```python
from build123d import *

# Parameters (mm, degrees)
SKETCH1_W           = 60
SKETCH1_H           = 7.9
BOSS_EXTRUDE1_DEPTH = 0.5
SKETCH2_W           = 2.6
SKETCH2_H           = 2.4
CUT_EXTRUDE1_DEPTH  = 61.519914078
LPATTERN1_COUNT     = 11
LPATTERN1_PITCH     = 5


with BuildPart() as part:
    # Sketch1 → Boss-Extrude1 (new body)
    with BuildSketch(Plane.XY):
        with Locations((30, -3.95)):
            Rectangle(SKETCH1_W, SKETCH1_H)
    extrude(amount=BOSS_EXTRUDE1_DEPTH)

    # Sketch2 → Cut-Extrude1 (cut, symmetric)
    with BuildSketch(Plane.XY.offset(0.5)):
        with Locations((3.8, -3.8)):
            Rectangle(SKETCH2_W, SKETCH2_H)
    cut_extrude1 = extrude(amount=CUT_EXTRUDE1_DEPTH, both=True, mode=Mode.SUBTRACT)

    # LPattern1: Cut-Extrude1 ×11
    with Locations(*[(i * LPATTERN1_PITCH, 0, 0) for i in range(1, LPATTERN1_COUNT)]):
        add(cut_extrude1, mode=Mode.SUBTRACT)


solid = part.part
```
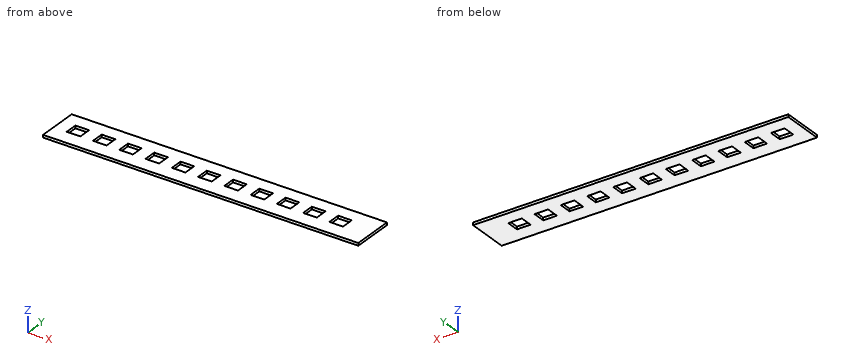
Model file for the job. Use its own axes, mm. Coordinates: 2 decimals unless noted, no trailing zeros. Loops run counter-clockwise (first coordinate to the right, second up) from the corner with the lowest first, then second, coordinate; pieces in that order, holes last. Notation, with made-up numbers: (-37, -8) - (-12, -8) arc R21 cw to (-12, 28) - close; hole circle Ø8 at (42, -10). An arc over 180 degrees is marked (long way). Answer as a JSON object with one key per item and string values. Group by question number.
(1) Probe line 1 along Y through (x, z) = (44, 0.4). List the from-to ranges inside material, lowest first.
(2) Cut at B-B (z = 0.3). State how many separate pieces and enclosed holes the cut face has, then the cut area to 3 significant figures.
(3) Cut at A-A (x = 9). Give the cut face in (y, z).
Geometry says:
{
 "1": {"line 1": "y = -7.9 to -5, -2.6 to 0"},
 "2": {"separate pieces": "1", "enclosed holes": "11", "area": "405 mm^2"},
 "3": {"outline": "(-7.9, 0) - (-5, 0) - (-5, 0.5) - (-7.9, 0.5) - close; (-2.6, 0) - (0, 0) - (0, 0.5) - (-2.6, 0.5) - close"}
}
